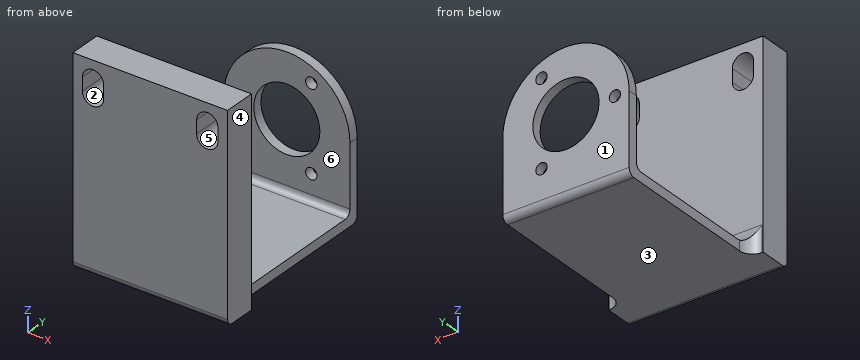
```python
from build123d import *

# Parameters (mm, degrees)
SKETCH_R     = 10.125
SKETCH_R_2   = 1.75
PAD_DEPTH    = 3
SKETCH001_W  = 38.7
SKETCH001_H  = 3
PAD001_DEPTH = 60
SKETCH002_W  = 47.4
SKETCH002_H  = 10
PAD002_DEPTH = 62
POCKET_DEPTH = 10
FILLET_R     = 2
FILLET001_R  = 5
FILLET002_R  = 2
FILLET003_R  = 4


with BuildPart() as part:
    # Sketch → Pad (new body)
    with BuildSketch(Plane.XZ):
        with BuildLine():
            ThreePointArc((19.35, -3e-06), (0, 19.35), (-19.35, -3e-06))
            Line((-19.35, -3e-06), (-19.35, -24.000003))
            Line((-19.35, -24.000003), (19.35, -24.000003))
            Line((19.35, -24.000003), (19.35, -3e-06))
        make_face()
        Circle(SKETCH_R, mode=Mode.SUBTRACT)
        with Locations((7.500003, 12.990379)):
            Circle(SKETCH_R_2, mode=Mode.SUBTRACT)
        with Locations((-15, 5e-06)):
            Circle(SKETCH_R_2, mode=Mode.SUBTRACT)
        with Locations((7.499994, -12.990384)):
            Circle(SKETCH_R_2, mode=Mode.SUBTRACT)
    extrude(amount=PAD_DEPTH)

    # Sketch001 (on Face9 of Pad) → Pad001 (join)
    with BuildSketch(Plane(origin=(0, 0, 0), x_dir=(1, 0, 0), z_dir=(0, 1, 0))):
        with Locations((0, 22.500003)):
            Rectangle(SKETCH001_W, SKETCH001_H)
    extrude(amount=-PAD001_DEPTH)

    # Sketch002 (on Face12 of Pad001) → Pad002 (join)
    with BuildSketch(Plane(origin=(0, 0, -24.000003), x_dir=(1, 0, 0), z_dir=(0, 0, -1))):
        with Locations((0, 55)):
            Rectangle(SKETCH002_W, SKETCH002_H)
    extrude(amount=-PAD002_DEPTH)

    # Sketch003 (on Face16 of Pad002) → Pocket (cut)
    with BuildSketch(Plane.XZ.offset(60)):
        with BuildLine():
            ThreePointArc((-14.25, 32), (-17.5, 35.25), (-20.75, 32))
            Line((-20.75, 32), (-20.75, 28))
            ThreePointArc((-20.75, 28), (-17.5, 24.75), (-14.25, 28))
            Line((-14.25, 32), (-14.25, 28))
        make_face()
        with BuildLine():
            ThreePointArc((20.75, 32), (17.5, 35.25), (14.25, 32))
            Line((14.25, 32), (14.25, 28))
            ThreePointArc((14.25, 28), (17.5, 24.75), (20.75, 28))
            Line((20.75, 32), (20.75, 28))
        make_face()
    extrude(amount=-POCKET_DEPTH, mode=Mode.SUBTRACT)

    # Fillet
    fillet_edges = [part.edges().sort_by_distance(p)[0] for p in [
        (0, 0, -24.000003),
        (0, -3, -21.000003),
    ]]
    fillet(fillet_edges, radius=FILLET_R)

    # Fillet001
    fillet001_edges = [part.edges().sort_by_distance(p)[0] for p in [
        (0, -50, -21.000003),
    ]]
    fillet(fillet001_edges, radius=FILLET001_R)

    # Fillet002
    fillet002_edges = [part.edges().sort_by_distance(p)[0] for p in [
        (0, -60, -24.000003),
    ]]
    fillet(fillet002_edges, radius=FILLET002_R)

    # Fillet003
    fillet003_edges = [part.edges().sort_by_distance(p)[0] for p in [
        (-19.35, -50, -22.500003),
        (-19.35, -50, -18.500003),
        (19.35, -50, -22.500003),
        (19.35, -50, -18.500003),
    ]]
    fillet(fillet003_edges, radius=FILLET003_R)


solid = part.part
```
Check sheet for the modelled part. Datum: model origin and axes. Units: mm. Face numbers are marked on the shaded views. A direction names the side the tool comes from. Give positions to 0.01 mm unless a question says otherwise; leave off trailing zeros. Order: outer loops, then holes, each group sorted by start corner. A loop starts at its lowest first (then second) coordinate and runs counter-clockwise, first axis right, second up. Notation, with made-up numbers: M 35.25,-17 L 53.25,-17 A27 ccw 53.25,11 Z; hole C 60.25,89 d9. An arc over 180 degrees is marked long. Answer in a Markdown table with one row per item.
1) Thickness scan on L1, parallel to Y at x = 7, z = -8.5; L2, parallel to Z at x = -13, y = -26.5; L3, parallel to Y at x = 22, z = 12.5. Record the ranges inside material, lowest first. Write a range as [from, to].
Filled sheet:
| item | result |
|---|---|
| L1 | y = [-60, -50], [-3, 0] |
| L2 | z = [-24, -21] |
| L3 | y = [-60, -50] |
2) Cross-section at C-C, the plane z = 27. Enter the section's corners in (x, y).
Filled sheet:
| item | result |
|---|---|
| outline | M -23.7,-60 L -20.59,-60 L -20.59,-50 L -23.7,-50 Z; M -14.41,-60 L 14.41,-60 L 14.41,-50 L -14.41,-50 Z; M 20.59,-60 L 23.7,-60 L 23.7,-50 L 20.59,-50 Z |
3) Cross-section at D-D, the plane x = 1.5. Enter the section's corners in (y, z), plus the area to 3 significant figures.
Filled sheet:
| item | result |
|---|---|
| outline | M -60,-22 A2 ccw -58,-24 L -2,-24 A2 ccw 0,-22 L 0,-10.01 L -3,-10.01 L -3,-19 A2 cw -5,-21 L -45,-21 A5 cw -50,-16 L -50,38 L -60,38 Z; M -3,10.01 L 0,10.01 L 0,19.29 L -3,19.29 Z |
| area | 835 mm2 |
4) Cross-section at B-B, the plane y = -56. Enter the section's corners in (x, z).
Filled sheet:
| item | result |
|---|---|
| outline | M -23.7,-24 L 23.7,-24 L 23.7,38 L -23.7,38 Z; hole M -20.75,28 A3.25 ccw -14.25,28 L -14.25,32 A3.25 ccw -20.75,32 Z; hole M 14.25,28 A3.25 ccw 20.75,28 L 20.75,32 A3.25 ccw 14.25,32 Z |
5) Access from +Z, -Z, +X, -X, +Y, -Y to the whole of each face (thin tool, end or side, straight path). Record for the marked faces 4, 5 and 6.
Filled sheet:
| item | result |
|---|---|
| face 4 | +Z, -Z, +X, +Y, -Y |
| face 5 | +Y, -Y |
| face 6 | +Z, +X, -X |
6) Cross-section at A-A, the plane x = 16. Enter the section's corners in (y, z), plus the area to 3 significant figures.
Filled sheet:
| item | result |
|---|---|
| outline | M -60,-22 A2 ccw -58,-24 L -2,-24 A2 ccw 0,-22 L 0,10.88 L -3,10.88 L -3,-19 A2 cw -5,-21 L -45,-21 A5 cw -50,-16 L -50,25.12 L -60,25.12 Z; M -60,34.88 L -50,34.88 L -50,38 L -60,38 Z |
| area | 772 mm2 |
7) Release check for a two-part mould opening along Z. For the marked faces 1, 2 and 3 record: +Z half, -Z half, draft (parallel to the pull), parting line (faces both ways), or undercut.
Filled sheet:
| item | result |
|---|---|
| face 1 | draft |
| face 2 | undercut |
| face 3 | -Z half |
8) Gauge pin test, flat ends, axial feed: P1, Ø5, axis at x = -5.5, y = -48.5, coming from the +Z side; P2, Ø19.5, axis at x = 0, y = -33, coming from the +Z side. Record the tip position at first contact, or that the pin passes through.
Filled sheet:
| item | result |
|---|---|
| P1 | stops at z = 38 |
| P2 | stops at z = -21 |
